Autodesk Inventor part; units mm, degrees
ref_plane "YZ Plane" through (0, 0, 0) normal (1, 0, 0) x (0, 1, 0)
ref_plane "XZ Plane" through (0, 0, 0) normal (0, 1, 0) x (-1, 0, 0)
ref_plane "XY Plane" through (0, 0, 0) normal (0, 0, 1) x (1, 0, 0)
sketch "スケッチ2" plane through (0, 0, 0) normal (1, 0, 0) x (0, 1, 0)
  circle A0 centre (0, 0) radius 6.25
  line L0 (13, 0) -> (-13, 0) construction
  line L1 (-13, 0) -> (-13, -24)
  line L2 (-13, -24) -> (13, -24)
  line L3 (13, -24) -> (13, 0)
  line L4 (13, -24) -> (16, -24)
  line L5 (16, -24) -> (16, -14.5)
  line L6 (16, -14.5) -> (13, -14.5)
  line L7 (13, -14.5) -> (13, -24)
  line L8 (13, 0) -> (-13, 0)
  line L9 (-13, 0) -> (-13, 3)
  line L10 (-13, 3) -> (13, 3)
  line L11 (13, 3) -> (13, 0)
  point P0 (13, 0)
  point P1 (5.4829, 3)
  point P2 (-5.4829, 3)
  point P3 (-13, 0)
  dimension "d0" = 12.5
  dimension "d1" = 26
  dimension "d2" = 24
  dimension "d3" = 3
  dimension "d4" = 9.5
  dimension "d5" = 3
extrude "プレート1" add sketch "スケッチ2" along normal blind 1.5 contours L8 L3 L2 L1 A0 | A0 L10 L11 L8 | L8 L9 L10 A0 | L6 L5 L4 L3
sketch "スケッチ3" plane through (1.5, 14.5, -24) normal (0, 1, 0) x (-1, 0, 0)
  line L0 (0, 9.5) -> (0, 0)
  line L1 (0, 0) -> (9.5, 0)
  line L2 (9.5, 0) -> (9.5, 9.5)
  line L3 (9.5, 9.5) -> (0, 9.5)
edge flange "フランジ1" height 9.5 angle 90 thickness 1.5 bend radius 1.5 thickness toward (0, 1, 0) relief tear relief width 1.5 relief depth 0.75 edges at (0, 16, -19.25) wall of the first edge with corners at (1.5, 14.5, -14.5) (1.5, 14.5, -24) (-8, 14.5, -24) (-8, 14.5, -14.5)
bend "曲げ1"
corner "コーナー1"
equation "\"d6\" = Thickness"
equation "\"d7\" = BendReliefWidth"
equation "\"d8\" = BendReliefDepth"
equation "\"d9\" = MinimumRemnant"
equation "\"d10\" = TransitionRadius"
equation "\"d13\" = BendRadius"
equation "\"d14\" = CornerReliefSize"
equation "\"d15\" = GapSize"
equation "\"d16\" = JacobiRadiusSize"
equation "\"BendRadius\" = Thickness"
equation "\"BendReliefWidth\" = Thickness"
equation "\"BendReliefDepth\" = 0.5 * Thickness"
equation "\"CornerReliefSize\" = 4 * Thickness"
equation "\"MinimumRemnant\" = 2 * Thickness"
equation "\"TransitionRadius\" = BendRadius"
equation "\"JacobiRadiusSize\" = BendRadius"
equation "\"GapSize\" = Thickness"
properties part number "hipjoint_toleg_under_down_right"
Design review of the part built by this model. Coordinates are the model's own, in mm. A direction names the side the tool comes from. Coordinates: 2 decimals unless noted, no trailing zeros. Loops run counter-clockwise (first coordinate to the right, second up) from the corner with the lowest first, then second, coordinate; pieces in that order, holes last. Notation, with made-up numbers: (-21.5, 26.5) -> (-9.5, 26.5) arc R9 cw to (-9.5, 39.5) -> close; hole circle Ø10 at (45.25, 16). An arc over 180 degrees is marked (long way). Use a Markdown table: item, result. Add a question column.
Item 1: Machinability: for faces 1 (the flat face through (1, 13, -6)), 2 (the flat face through (-5, 14.5, -19)), 3 (the cylindrical face through (0.6, 15.14, -19.32)), which of the approach directions +Z, -Z, +X, -X, +Y, -Y give a long, thin tool a straight path to every point of the face, cutting with its end or side? Answer none if there is none.
Item 2: We need section B-B, the plane x = 0.5. Write out the cut boundary in (y, z), and give its area (3 significant figures).
Item 3: We need section D-D, the plane y = 0. Write out the cut boundary in (x, z).
Item 4: We need section C-C, the plane z = -16.25. Write out the cut boundary in (x, y), and give its area (3 significant figures).
Item 5: We need section A-A, the plane z = 0. Write out the cut boundary in (x, y), and give its area (4 significant figures).
Item 6: Clearance check with a flat-ended pin moving along its axis: P1, Ø0.9, axis at x = -3, y = 14.5, coming from the +Z side. State where the tip first meets the part, or that it passes through.
Item 7: Wall thickness on L1, parallel to Y at x = 1.1, z = 0; L2, parallel to X at y = -0.75, z = -8; L3, parallel to Z at x = 0.7, y = 0: over which ranges is each line inside the solid? List them lowest first. Write a range as from..to.
Numbers:
| question | item | result |
|---|---|---|
| 1 | face 1 | +Z, +X, -X, +Y |
| 1 | face 2 | +Z, -Z, -X, -Y |
| 1 | face 3 | +Z, -Z, +X, +Y |
| 2 | outline | (-13, -24) -> (15.24, -24) -> (15.24, -14.5) -> (13, -14.5) -> (13, 3) -> (5.48, 3) arc R6.25 cw (long way) to (-5.48, 3) -> (-13, 3) -> close |
| 2 | area | 626 mm^2 |
| 3 | outline | (0, -24) -> (1.5, -24) -> (1.5, -6.25) -> (0, -6.25) -> close |
| 4 | outline | (-8, 14.5) -> (-1.5, 14.5) arc R1.5 cw to (0, 13) -> (0, -13) -> (1.5, -13) -> (1.5, 13) arc R3 ccw to (-1.5, 16) -> (-8, 16) -> close |
| 4 | area | 54.1 mm^2 |
| 5 | outline | (0, -13) -> (1.5, -13) -> (1.5, -6.25) -> (0, -6.25) -> close; (0, 6.25) -> (1.5, 6.25) -> (1.5, 13) -> (0, 13) -> close |
| 5 | area | 20.25 mm^2 |
| 6 | P1 | stops at z = -14.5 |
| 7 | L1 | y = -13..-6.25, 6.25..13 |
| 7 | L2 | x = 0..1.5 |
| 7 | L3 | z = -24..-6.25 |
